For this review, take the finished solid that the model builds, in its own axes (mm). A direction names the side the tool comes from. Give positions to 0.01 mm unless a question says otherwise; leave off trailing zeros. Order: outer loops, then holes, each group sorted by start corner. A loop starts at its lowest first (then second) coordinate and runs counter-clockwise, first axis right, second up.
from build123d import *

# Parameters (mm, degrees)
BOSS_EXTRUDE1_DEPTH = 8
CUT_EXTRUDE1_REACH  = 62.515
SKETCH3_R           = 1.3
CUT_EXTRUDE2_DEPTH  = 84.004180545
FILLET6_R           = 2
FILLET7_R           = 1
FILLET8_R           = 10
CUT_EXTRUDE3_REACH  = 62.515
SKETCH4_R           = 1.3


with BuildPart() as part:
    # Sketch1 → Boss-Extrude1 (new body)
    with BuildSketch(Plane(origin=(0, 0, 0), x_dir=(0, 1, 0), z_dir=(0, 0, 1))):
        Polygon((-56.323529412, 20.632352941), (-56.323529412, -11.367647059), (-51.323529412, -11.367647059), (-51.323529412, -3.367647059), (-31.323529412, -0.367647059), (-1.323529412, -0.367647059), (18.676470588, -3.367647059), (18.676470588, -11.367647059), (23.676470588, -11.367647059), (23.676470588, 20.632352941), (18.676470588, 20.632352941), (18.676470588, 12.632352941), (-1.323529412, 9.632352941), (-31.323529412, 9.632352941), (-51.323529412, 12.632352941), (-51.323529412, 20.632352941), align=None)
    extrude(amount=BOSS_EXTRUDE1_DEPTH)

    # Sketch2 → Cut-Extrude1 (cut, up to next)
    with BuildSketch(Plane.XY.offset(8), mode=Mode.PRIVATE) as cut_extrude1_sk1:
        Polygon((-7.632352941, -51.323529412), (-4.632352941, -31.323529412), (-1.632352941, -51.323529412), align=None)
    cut_extrude1_tool1 = extrude(cut_extrude1_sk1.sketch, amount=-CUT_EXTRUDE1_REACH, mode=Mode.PRIVATE) & part.part
    # Sketch2 → Cut-Extrude1 (cut, up to next)
    with BuildSketch(Plane.XY.offset(8), mode=Mode.PRIVATE) as cut_extrude1_sk2:
        Polygon((-1.632352941, 18.676470588), (-7.632352941, 18.676470588), (-4.632352941, -1.323529412), align=None)
    cut_extrude1_tool2 = extrude(cut_extrude1_sk2.sketch, amount=-CUT_EXTRUDE1_REACH, mode=Mode.PRIVATE) & part.part
    add(cut_extrude1_tool1.solids().sort_by_distance((-4.632353, -44.656863, 8))[0], mode=Mode.SUBTRACT)
    add(cut_extrude1_tool2.solids().sort_by_distance((-4.632353, 12.009804, 8))[0], mode=Mode.SUBTRACT)

    # Sketch3 → Cut-Extrude2 (cut, through all)
    with BuildSketch(Plane.XZ.offset(56.323529412)):
        with Locations(Location((-17.132352941, 4, 0), (0, 0, 270))):
            Circle(SKETCH3_R)
        with Locations(Location((7.867647059, 4, 0), (0, 0, 270))):
            Circle(SKETCH3_R)
    extrude(amount=-CUT_EXTRUDE2_DEPTH, mode=Mode.SUBTRACT)

    # Fillet6
    fillet6_edges = [part.edges().sort_by_distance(p)[0] for p in [
        (-12.632352941, -51.323529412, 4),
        (-12.632352941, 18.676470588, 4),
        (3.367647059, 18.676470588, 4),
        (3.367647059, -51.323529412, 4),
    ]]
    fillet(fillet6_edges, radius=FILLET6_R)

    # Fillet7
    fillet7_edges = [part.edges().sort_by_distance(p)[0] for p in [
        (-1.632352941, -51.323529412, 4),
        (-7.632352941, -51.323529412, 4),
        (-4.632352941, -31.323529412, 4),
        (-1.632352941, 18.676470588, 4),
        (-4.632352941, -1.323529412, 4),
        (-7.632352941, 18.676470588, 4),
    ]]
    fillet(fillet7_edges, radius=FILLET7_R)

    # Fillet8
    fillet8_edges = [part.edges().sort_by_distance(p)[0] for p in [
        (-9.632352941, -31.323529412, 4),
        (-9.632352941, -1.323529412, 4),
        (0.367647059, -1.323529412, 4),
        (0.367647059, -31.323529412, 4),
    ]]
    fillet(fillet8_edges, radius=FILLET8_R)

    # Sketch4 → Cut-Extrude3 (cut, up to next)
    with BuildSketch(Plane.XY.offset(8), mode=Mode.PRIVATE) as cut_extrude3_sk1:
        with Locations((-4.632352941, -8.323529412)):
            Circle(SKETCH4_R)
    cut_extrude3_tool1 = extrude(cut_extrude3_sk1.sketch, amount=-CUT_EXTRUDE3_REACH, mode=Mode.PRIVATE) & part.part
    # Sketch4 → Cut-Extrude3 (cut, up to next)
    with BuildSketch(Plane.XY.offset(8), mode=Mode.PRIVATE) as cut_extrude3_sk2:
        with Locations((-4.632352941, -24.323529412)):
            Circle(SKETCH4_R)
    cut_extrude3_tool2 = extrude(cut_extrude3_sk2.sketch, amount=-CUT_EXTRUDE3_REACH, mode=Mode.PRIVATE) & part.part
    add(cut_extrude3_tool1.solids().sort_by_distance((-4.632353, -8.323529, 8))[0], mode=Mode.SUBTRACT)
    add(cut_extrude3_tool2.solids().sort_by_distance((-4.632353, -24.323529, 8))[0], mode=Mode.SUBTRACT)


solid = part.part
1) Tool access review of faces 4 (the face through (-5, -26, 0)), 5 (the face through (-4.652, -37.065, 3.944)), 6 (the face through (-9.66, -1.34, 4.06)), 7 (the face through (9, 18.676, 3)): name each direction out of +Z, -Z, +X, -X, +Y, -Y from which nothing blocks a thin tool from reaching the whole face with its end or side.
Answer sheet:
face 4: -Z, +X, -X, +Y, -Y
face 5: +Z, -Z
face 6: +Z, -Z, -X
face 7: +Z, -Z, +X
2) We need section C-C on y = -29. Give the boundary of the cut face in (x, z), then the cut area to 3 significant figures.
Answer sheet:
outline: (-9.63, 0) - (0.37, 0) - (0.37, 8) - (-9.63, 8) - close
area: 80.0 mm2
3) To check wall thickness, follow line 1 (X direction, y = -52.7, z = 4); line 2 (Y direction, x = -4.5, z = 7.25); line 3 (Y direction, x = -17.5, z = 7.5). State the ranges of each line that lie inside material, in increasing order.
Answer sheet:
line 1: x = -20.63 to -18.43, -15.83 to 6.57, 9.17 to 11.37
line 2: y = -56.32 to -51.32, -37.07 to -25.62, -23.03 to -9.62, -7.03 to 4.43, 18.68 to 23.68
line 3: y = -56.32 to -51.32, 18.68 to 23.68
4) Draft analysis for pull direction X (two halves, no side actions). For faces 1 (the face through (6.6, -53.86, 4.28)), 2 (the face through (-20.632, 21, 4)), 3 (the face through (0.368, -17, 4)), state which applies: +X half, -X half, draft (parallel to the pull), parting line (faces both ways), or undercut.
Answer sheet:
face 1: undercut
face 2: -X half
face 3: +X half
5) Clearance check with flat-ended pins moving along their axes: pin 1 (2 mm diameter, centred on x = 8, z = 4, fed in from -Y); pin 2 (2.5 mm diameter, centred on y = -15, z = 4, fed in from +X); pin 3 (2 mm diameter, centred on y = 6.5, z = 4, fed in from -X); pin 4 (2.5 mm diameter, centred on y = -14, z = 3.5, fed in from -X). State where each tip first meets the part, or that it passes through.
Answer sheet:
pin 1: passes through
pin 2: stops at x = 0.37
pin 3: stops at x = -10.96
pin 4: stops at x = -9.63
6) We need section A-A on y = -44. Give the boundary of the cut face in (x, z).
Answer sheet:
outline: (-11.53, 0) - (-6.53, 0) - (-6.53, 8) - (-11.53, 8) - close; (-2.73, 0) - (2.27, 0) - (2.27, 8) - (-2.73, 8) - close
7) We need section B-B on z = 4. Count the separate pieces of the cut face and the enclosed holes in it, then the cut area to 3 significant figures.
Answer sheet:
separate pieces: 5
enclosed holes: 4
area: 972 mm2
